```python
from build123d import *

# Parameters (mm, degrees)
F1_DEPTH = 12
F2_R     = 1
F3_W     = 3.8
F3_H     = 3.8
F4_DEPTH = 2.3
F5_R     = 1.182199
F6_DEPTH = 1.2


with BuildPart() as f1:
    # F0 (on Front) → F1 (new body)
    with BuildSketch(Plane.XZ):
        with BuildLine():
            Line((17.5, 29.8), (-17.5, 29.8))
            ThreePointArc((-17.5, 29.8), (-21.035534, 28.335534), (-22.5, 24.8))
            Line((-22.5, 24.8), (-22.5, -24.8))
            ThreePointArc((-22.5, -24.8), (-21.035534, -28.335534), (-17.5, -29.8))
            Line((-17.5, -29.8), (17.5, -29.8))
            ThreePointArc((17.5, -29.8), (21.035534, -28.335534), (22.5, -24.8))
            Line((22.5, -24.8), (22.5, 24.8))
            ThreePointArc((22.5, 24.8), (21.035534, 28.335534), (17.5, 29.8))
        make_face()
    extrude(amount=F1_DEPTH)

    # F2
    f2_edges = [f1.edges().sort_by_distance(p)[0] for p in [
        (0, -12, 29.8),
        (-21.035534, -12, 28.335534),
        (-22.5, -12, 0),
        (-21.035534, -12, -28.335534),
        (0, -12, -29.8),
        (21.035534, -12, -28.335534),
        (22.5, -12, 0),
        (21.035534, -12, 28.335534),
    ]]
    fillet(f2_edges, radius=F2_R)

    # F3 (on face) → F4 (cut)
    with BuildSketch(Plane(origin=(0, 0, 0), x_dir=(-1, 0, 0), z_dir=(0, 1, 0))):
        with Locations((10, 20)):
            Rectangle(F3_W, F3_H)
        with Locations((-14, 0)):
            Rectangle(F3_W, F3_H)
        with Locations((10, -20)):
            Rectangle(F3_W, F3_H)
    extrude(amount=-F4_DEPTH, mode=Mode.SUBTRACT)

    # F5 (on face) → F6 (join)
    with BuildSketch(Plane.XZ.offset(12)):
        with Locations((-15, 23.5)):
            Circle(F5_R)
        with Locations((-15, 17.5)):
            Circle(F5_R)
        with Locations((-15, 11.5)):
            Circle(F5_R)
        with Locations((-15, 5.5)):
            Circle(F5_R)
        with Locations((-15, -0.5)):
            Circle(F5_R)
        with Locations((-9, 23.5)):
            Circle(F5_R)
        with Locations((-9, 17.5)):
            Circle(F5_R)
        with Locations((-9, 11.5)):
            Circle(F5_R)
        with Locations((-9, 5.5)):
            Circle(F5_R)
        with Locations((-9, -0.5)):
            Circle(F5_R)
        with Locations((-3, 23.5)):
            Circle(F5_R)
        with Locations((-3, 17.5)):
            Circle(F5_R)
        with Locations((-3, 11.5)):
            Circle(F5_R)
        with Locations((-3, 5.5)):
            Circle(F5_R)
        with Locations((-3, -0.5)):
            Circle(F5_R)
        with Locations((3, 23.5)):
            Circle(F5_R)
        with Locations((3, 17.5)):
            Circle(F5_R)
        with Locations((3, 11.5)):
            Circle(F5_R)
        with Locations((3, 5.5)):
            Circle(F5_R)
        with Locations((3, -0.5)):
            Circle(F5_R)
        with Locations((-15, -6.5)):
            Circle(F5_R)
        with Locations((-15, -12.5)):
            Circle(F5_R)
        with Locations((-15, -18.5)):
            Circle(F5_R)
        with Locations((-15, -24.5)):
            Circle(F5_R)
        with Locations((-9, -6.5)):
            Circle(F5_R)
        with Locations((-9, -12.5)):
            Circle(F5_R)
        with Locations((-9, -18.5)):
            Circle(F5_R)
        with Locations((-9, -24.5)):
            Circle(F5_R)
        with Locations((-3, -6.5)):
            Circle(F5_R)
        with Locations((-3, -12.5)):
            Circle(F5_R)
        with Locations((-3, -18.5)):
            Circle(F5_R)
        with Locations((-3, -24.5)):
            Circle(F5_R)
        with Locations((3, -6.5)):
            Circle(F5_R)
        with Locations((3, -12.5)):
            Circle(F5_R)
        with Locations((3, -18.5)):
            Circle(F5_R)
        with Locations((3, -24.5)):
            Circle(F5_R)
        with Locations((9, 23.5)):
            Circle(F5_R)
        with Locations((9, 17.5)):
            Circle(F5_R)
        with Locations((9, 11.5)):
            Circle(F5_R)
        with Locations((9, 5.5)):
            Circle(F5_R)
        with Locations((9, -0.5)):
            Circle(F5_R)
        with Locations((9, -6.5)):
            Circle(F5_R)
        with Locations((9, -12.5)):
            Circle(F5_R)
        with Locations((9, -18.5)):
            Circle(F5_R)
        with Locations((9, -24.5)):
            Circle(F5_R)
        with Locations((15, 23.5)):
            Circle(F5_R)
        with Locations((15, 17.5)):
            Circle(F5_R)
        with Locations((15, 11.5)):
            Circle(F5_R)
        with Locations((15, 5.5)):
            Circle(F5_R)
        with Locations((15, -0.5)):
            Circle(F5_R)
        with Locations((15, -6.5)):
            Circle(F5_R)
        with Locations((15, -12.5)):
            Circle(F5_R)
        with Locations((15, -18.5)):
            Circle(F5_R)
        with Locations((15, -24.5)):
            Circle(F5_R)
    extrude(amount=F6_DEPTH)


solid = f1.part
```
Here's how the part is built. I have some questions about the finished solid (model axes, mm). A direction names the side the tool comes from. Give positions to 0.01 mm unless a question says otherwise; leave off trailing zeros. Loops run counter-clockwise (first coordinate to the right, second up) from the corner with the lowest first, then second, coordinate; pieces in that order, holes last. Notation, with made-up numbers: M 32,27 L 91,27 A23 ccw 91,47 Z; hole C 88.5,64 d5. An arc over 180 degrees is marked long. Use one line per item in the form item = value. Start each with the question number.
Q1. Which directions (+Z, -Z, +X, -X, +Y, -Y) give clear straight access to the entire face, cutting with the end or side of a thin tool? Please do faces 4 (the cylindrical face through (-4.18, -12.59, -18.45)), 5 (the flat face through (15, -13.2, 24)), 6 (the flat face through (-10, -1, 21.9)).
Q2. I need wall thicknesses on line 1 along Z through (x, y) = (13, -0.25); line 2 along Y through (x, z) = (11, 13.5); line 3 along Z through (x, y) = (18, -5.5). Which ranges of each line are inside material? Lowest first, please.
Q3. If we section it at A-A (y = -1): Write out the boundary of the cut face in (x, z).
Q4. If we section it at C-C (x = 0): Write out the boundary of the cut face in (y, z), then the cut area to 3 significant figures.
Q5. Thinking about a two-plate mould opening in X: for faces 1 (the cylindrical face through (-15.87, -12.59, -11.7)), 2 (the flat face through (0, -5, 29.8)), 3 (the flat face through (-10, -1, 18.1)), which applies, +X half, -X half, draft (parallel to the pull), parting line (faces both ways), or undercut?
Q6. Will these pins go through, and if not, where does the flat tip stop? pin 1 Ø1.1 at (x, z) = (14.5, 0) entering from +Y; pin 2 Ø4 at (x, z) = (-17, -9.5) entering from -Y.
Taken from the geometry:
q1.face_4 = -Y
q1.face_5 = +Z, -Z, +X, -X, -Y
q1.face_6 = +Y
q2.line_1 = -29.8 to -1.9, 1.9 to 29.8
q2.line_2 = -12 to 0
q2.line_3 = -29.77 to 29.77
q3.outline = M -22.5,-24.8 A5 ccw -17.5,-29.8 L 17.5,-29.8 A5 ccw 22.5,-24.8 L 22.5,24.8 A5 ccw 17.5,29.8 L -17.5,29.8 A5 ccw -22.5,24.8 Z; hole M -11.9,-21.9 L -8.1,-21.9 L -8.1,-18.1 L -11.9,-18.1 Z; hole M -11.9,18.1 L -8.1,18.1 L -8.1,21.9 L -11.9,21.9 Z; hole M 12.1,-1.9 L 15.9,-1.9 L 15.9,1.9 L 12.1,1.9 Z
q4.outline = M -12,-28.8 A1 ccw -11,-29.8 L 0,-29.8 L 0,29.8 L -11,29.8 A1 ccw -12,28.8 Z
q4.area = 715 mm^2
q5.face_1 = undercut
q5.face_2 = draft
q5.face_3 = undercut
q6.pin_1 = -2.3
q6.pin_2 = -12
